from build123d import *

# Parameters (mm, degrees)
SKETCH1_W           = 35
SKETCH1_H           = 45
BOSS_EXTRUDE1_DEPTH = 125
SKETCH2_W           = 35
SKETCH2_H           = 41
CUT_EXTRUDE1_DEPTH  = 36


with BuildPart() as part:
    # Sketch1 → Boss-Extrude1 (new body)
    with BuildSketch(Plane.XY):
        Rectangle(SKETCH1_W, SKETCH1_H)
    extrude(amount=BOSS_EXTRUDE1_DEPTH)

    # Sketch2 → Cut-Extrude1 (cut, through all)
    with BuildSketch(Plane.ZY.offset(17.5)):
        with Locations((107.5, 0)):
            Rectangle(SKETCH2_W, SKETCH2_H)
    extrude(amount=-CUT_EXTRUDE1_DEPTH, mode=Mode.SUBTRACT)


solid = part.part
Model file for the job. Use its own axes, mm. A direction names the side the tool comes from. Coordinates: 2 decimals unless noted, no trailing zeros. Write each loop counter-clockwise with the first axis right and the second up, starting at its lowest first coordinate (ties: lowest second). Pieces come first, ordered by that corner, then holes. Notation, with made-up numbers: (-30.5, 81.5) -> (-24.5, 81.5) arc R19 ccw to (-24.5, 95.5) -> close; hole circle Ø2 at (68.25, 40.25). An arc over 180 degrees is marked (long way). One line per item, written item: value. Start each with the question number.
1) Probe probe 1 along Y at (x, z) = (-1, 117); probe 2 along Z at (x, y) = (-8.5, 1.5). List the from-to ranges inside material, lowest first.
2) Flat gauge pin, fed straight in: pin 1 Ø4 at (x, y) = (9.5, 0) entering from +Z. Where does the tip first touch, or does it go through?
3) Which spindle directions (+Z, -Z, +X, -X, +Y, -Y) get a long thin tool onto all of the face, cutting with end or side? Do faces 1 (the face through (0, 20.5, 107)), 2 (the face through (17.5, 0, 48)). Say none if no direction does.
4) Slice it at C-C on y = -7.5. Write the cut outline in (x, z), then the cut area to 3 significant figures.
5) Slice it at B-B on x = 4. Write the cut outline in (y, z), then the cut area to 3 significant figures.
6) Slice it at A-A on z = 95. Write the cut outline in (x, y).
7) Pull direction Y, two halves, no side cores. Call faces 3 (the face through (-17.5, 0, 48)), 4 (the face through (0, 0, 90)), 5 (the face through (0, 22.5, 62)), 6 (the face through (0, -22.5, 62)): +Y half, -Y half, draft (parallel to the pull), parting line (faces both ways), or undercut.
Answers follow:
1. probe 1: -22.5 to -20.5, 20.5 to 22.5
1. probe 2: 0 to 90
2. pin 1: z = 90
3. face 1: +Z, +X, -X
3. face 2: +Z, -Z, +X, +Y, -Y
4. outline: (-17.5, 0) -> (17.5, 0) -> (17.5, 90) -> (-17.5, 90) -> close
4. area: 3,150 mm2
5. outline: (-22.5, 0) -> (22.5, 0) -> (22.5, 125) -> (20.5, 125) -> (20.5, 90) -> (-20.5, 90) -> (-20.5, 125) -> (-22.5, 125) -> close
5. area: 4,190 mm2
6. outline: (-17.5, -22.5) -> (17.5, -22.5) -> (17.5, -20.5) -> (-17.5, -20.5) -> close; (-17.5, 20.5) -> (17.5, 20.5) -> (17.5, 22.5) -> (-17.5, 22.5) -> close
7. face 3: draft
7. face 4: undercut
7. face 5: +Y half
7. face 6: -Y half
